Input: dimensioned drawing with shaded views. Units: mm. Origin: part minimum x, y, z. Give positions to 0.01 mm unless a question says otherwise; leave off trailing zeros. Order: outer loops, then holes, each group sorted by start corner. A loop starts at its lowest first (then second) coordinate and runs counter-clockwise, first axis right, second up.
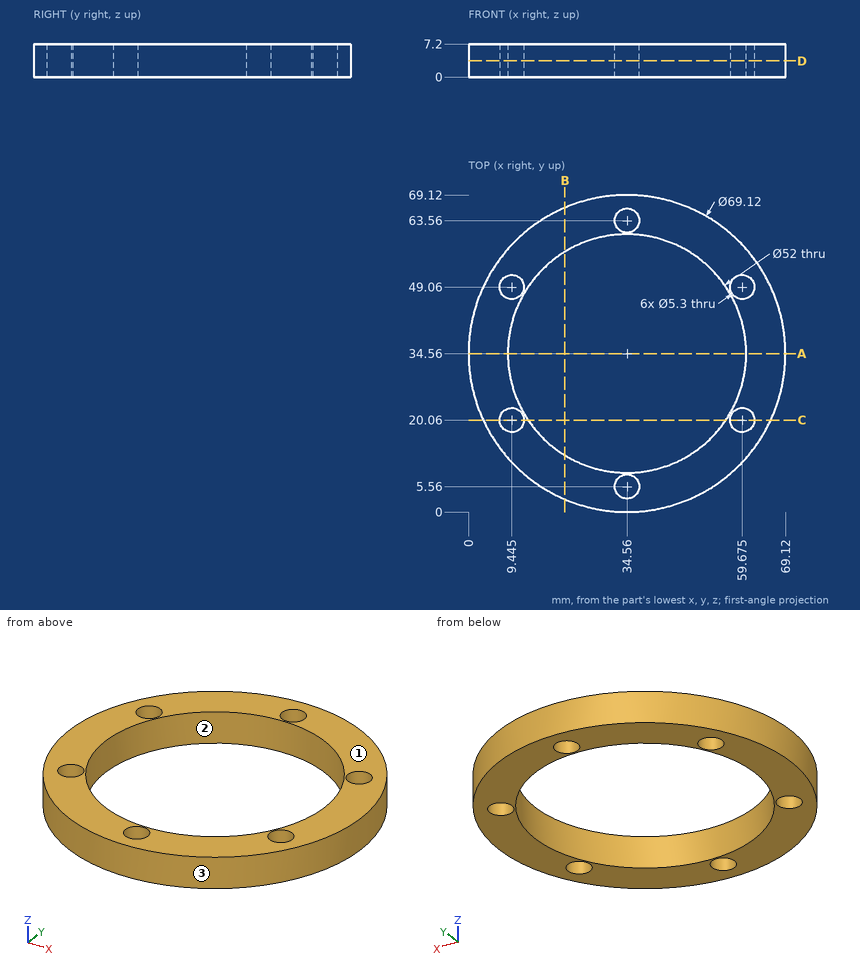
1) Section query B-B, the plane x = 21. Return the cut outline in (y, z), and give its area (3 significant figures).
Report:
outline: (2.77, 0) - (12.38, 0) - (12.38, 7.2) - (2.77, 7.2) - close; (56.74, 0) - (66.35, 0) - (66.35, 7.2) - (56.74, 7.2) - close
area: 138 mm2
2) Section query D-D, the plane z = 3.5. Count the separate pieces of the cut face and the enclosed holes in it, and give its area (3 significant figures).
Report:
separate pieces: 1
enclosed holes: 7
area: 1,500 mm2
3) Draft query along Y for the marked faces 1, 2 and 3. Return one class per face: +Y half, -Y half, draft (parallel to the pull), parting line (faces both ways), or undercut.
Report:
face 1: draft
face 2: undercut
face 3: parting line
4) Section query C-C, the plane y = 20.06. Return the cut outline in (x, z) (1 decimal).
Report:
outline: (3.2, 0) - (6.8, 0) - (6.8, 7.2) - (3.2, 7.2) - close; (12.1, 0) - (13, 0) - (13, 7.2) - (12.1, 7.2) - close; (56.1, 0) - (57, 0) - (57, 7.2) - (56.1, 7.2) - close; (62.3, 0) - (65.9, 0) - (65.9, 7.2) - (62.3, 7.2) - close
5) Material intervals for L1, parallel to Y at x = 34.56, z = 5; L2, parallel to X at y = 18, z = 4.5 (1 decimal); L3, parallel to X at y = 53.5, z = 6.5, sorted ascending.
Report:
L1: y = 0 to 2.91, 8.21 to 8.56, 60.56 to 60.91, 66.21 to 69.12
L2: x = 4.2 to 7.8, 11.1 to 14.5, 54.6 to 58, 61.3 to 64.9
L3: x = 5.65 to 16.75, 52.37 to 63.47
6) Pin query (flat end, axial travel): pin 1 (7 mm diameter, centred on x = 59.67, y = 20.06, fed in from -Z); pin 2 (3 mm diameter, centred on y = 14, z = 5.5, fed in from -X); pin 3 (3 mm diameter, centred on y = 27, z = 6.5, fed in from +X). Return the tip coordinate at first contact, or that it passes through.
Report:
pin 1: stops at z = 0
pin 2: stops at x = 5.73
pin 3: stops at x = 68.58
7) Section query A-A, the plane y = 34.56. Return the cut outline in (x, z), and give its area (3 significant figures).
Report:
outline: (0, 0) - (8.56, 0) - (8.56, 7.2) - (0, 7.2) - close; (60.56, 0) - (69.12, 0) - (69.12, 7.2) - (60.56, 7.2) - close
area: 123 mm2
